Autodesk Inventor part; units mm, degrees
ref_plane "YZ Plane" through (0, 0, 0) normal (1, 0, 0) x (0, 1, 0)
ref_plane "XZ Plane" through (0, 0, 0) normal (0, 1, 0) x (-1, 0, 0)
ref_plane "XY Plane" through (0, 0, 0) normal (0, 0, 1) x (1, 0, 0)
sketch "Sketch1" plane through (0, 0, 0) normal (0, 1, 0) x (-1, 0, 0)
  line L0 (-22.9214, -0.0293) -> (5.0786, -0.0293)
  circle A0 centre (5.0786, -0.0293) radius 2.5
  circle A1 centre (-22.9214, -0.0293) radius 2.5
  circle A2 centre (-22.9214, -0.0293) radius 5
  circle A3 centre (5.0786, -0.0293) radius 5
  line L1 (-8.9214, -0.0293) -> (-8.9214, -3.8509)
  line L2 (-8.9214, -3.8509) -> (-8.9214, -0.0293)
  line L3 (-8.9214, -0.0293) -> (-8.9214, 3.8269)
  arc A4 (-22.1098, 4.9044) -> (4.267, 4.9044) centre (-8.9214, 85.0769) ccw
  arc A5 (4.2428, -4.9589) -> (-22.0856, -4.9589) centre (-8.9214, -82.6063) ccw
  point P0 (0, 0)
  dimension "d0" = 28
  dimension "d1" = 5
  dimension "d2" = 5
  dimension "d3" = 10
  dimension "d4" = 10
extrude "Extrusion1" add sketch "Sketch1" along normal blind 5
properties part number "body-connector"
Input: part model. Units: mm. Frame: model coordinates. Give positions to 0.01 mm unless a question says otherwise; leave off trailing zeros. Write each loop counter-clockwise with the first axis right and the second up, starting at its lowest first coordinate (ties: lowest second). Pieces come first, ordered by that corner, then holes.
Q1. Section A-A, the plane x = -3.5. Output: boundary loops of the cut face in (y, z), plus the area to 3 significant figures.
Q2. Section D-D, the plane z = -0.5. Output: boundary loops of the cut face in (x, y), plus the area to 3 significant figures.
Q3. Section B-B, the plane z = 1. Output: boundary loops of the cut face in (x, y).
Q4. Material intervals for probe 1 along X at (y, z) = (1.9, 0); probe 2 along Z at (x, y) = (-5, 4); probe 3 along X at (y, z) = (0.25, 1.25), sorted ascending.
Q5. First-contact query: P1, Ø2, axis at y = 2, z = 3, coming from the -X side; P2, Ø3, axis at x = 22.92, z = -0.03, coming from the -Y side; P3, Ø6, axis at x = 9, z = 4, coming from the +Y side. Flat tips, straight axial feed; report the tip coordinate or a pass-through.
Q6. Section C-C, the plane y = 1.9. Output: boundary loops of the cut face in (x, z).
Q7. Pull-direction query (Z, two-part tool) for faces 1 (the face through (9.11, 2.46, -3.85)), 2 (the face through (9, 0, 0)), 3 (the face through (25.42, 2.46, -0.14)); classes: pulls with the +Z half, pulls with the -Z half, needs draft (parallel to the pull), parting line crosses it, or undercut.
Filled in:
1. outline: (0, -4.84) - (5, -4.84) - (5, -1.97) - (0, -1.97) - close; (0, 1.91) - (5, 1.91) - (5, 4.78) - (0, 4.78) - close
1. area: 28.7 mm2
2. outline: (-10.06, 0) - (-7.53, 0) - (-7.53, 5) - (-10.06, 5) - close; (-2.62, 0) - (20.47, 0) - (20.47, 5) - (-2.62, 5) - close; (25.38, 0) - (27.9, 0) - (27.9, 5) - (25.38, 5) - close
2. area: 141 mm2
3. outline: (-9.97, 0) - (-7.36, 0) - (-7.36, 5) - (-9.97, 5) - close; (-2.8, 0) - (20.64, 0) - (20.64, 5) - (-2.8, 5) - close; (25.2, 0) - (27.81, 0) - (27.81, 5) - (25.2, 5) - close
4. probe 1: x = -10.08 to -7.58, -2.58 to 20.42, 25.42 to 27.92
4. probe 2: z = -5.03 to -2.53, 2.47 to 4.97
4. probe 3: x = -9.91 to -7.23, -2.93 to 20.77, 25.07 to 27.75
5. P1: stops at x = -9.65
5. P2: passes through
5. P3: stops at y = 5
6. outline: (-4.27, 4.9) arc R5 ccw (long way) to (-4.24, -4.96) arc R78.76 cw to (22.09, -4.96) arc R5 ccw (long way) to (22.11, 4.9) arc R81.25 cw to start; hole circle Ø5 at (-5.08, -0.03); hole circle Ø5 at (22.92, -0.03)
7. face 1: pulls with the -Z half
7. face 2: needs draft
7. face 3: undercut
